from build123d import *

# Parameters (mm, degrees)
SK_TOP_PLATE_R         = 1.7
SK_TOP_PLATE_R_2       = 6
TOP_PLATE_DEPTH        = 10
SK_YAW_PILOT_RECESS_R  = 17.15
YAW_PILOT_RECESS_DEPTH = 2.2
SK_BACK_PLATE_W        = 132
SK_BACK_PLATE_H        = 100
SK_BACK_PLATE_R        = 2.25
SK_BACK_PLATE_R_2      = 13
BACK_PLATE_DEPTH       = 8
RIB_DEPTH              = 8


with BuildPart() as part:
    # SK_Top_Plate → Top_Plate (new body)
    with BuildSketch(Plane.XY.offset(72)):
        Polygon((-122, 45), (18, 45), (36, 27), (36, -27), (18, -45), (-122, -45), (-140, -27), (-140, 27), align=None)
        with Locations((23, 0)):
            Circle(SK_TOP_PLATE_R, mode=Mode.SUBTRACT)
        with Locations((11.5, -19.918584287)):
            Circle(SK_TOP_PLATE_R, mode=Mode.SUBTRACT)
        with Locations((-11.5, -19.918584287)):
            Circle(SK_TOP_PLATE_R, mode=Mode.SUBTRACT)
        with Locations((-23, 0)):
            Circle(SK_TOP_PLATE_R, mode=Mode.SUBTRACT)
        with Locations((-11.5, 19.918584287)):
            Circle(SK_TOP_PLATE_R, mode=Mode.SUBTRACT)
        with Locations((11.5, 19.918584287)):
            Circle(SK_TOP_PLATE_R, mode=Mode.SUBTRACT)
        Circle(SK_TOP_PLATE_R_2, mode=Mode.SUBTRACT)
    extrude(amount=TOP_PLATE_DEPTH)

    # SK_Yaw_Pilot_Recess → Yaw_Pilot_Recess (cut)
    with BuildSketch(Plane.XY.offset(82)):
        Circle(SK_YAW_PILOT_RECESS_R)
    extrude(amount=-YAW_PILOT_RECESS_DEPTH, mode=Mode.SUBTRACT)

    # SK_Back_Plate → Back_Plate (add)
    with BuildSketch(Plane(origin=(-140, 0, 0), x_dir=(0, 0, -1), z_dir=(1, 0, 0))):
        with Locations((-16, 0)):
            Rectangle(SK_BACK_PLATE_W, SK_BACK_PLATE_H)
        with Locations((39.726819898, -16.455387592)):
            Circle(SK_BACK_PLATE_R, mode=Mode.SUBTRACT)
        with Locations((16.455387592, -39.726819898)):
            Circle(SK_BACK_PLATE_R, mode=Mode.SUBTRACT)
        with Locations((-16.455387592, -39.726819898)):
            Circle(SK_BACK_PLATE_R, mode=Mode.SUBTRACT)
        with Locations((-39.726819898, -16.455387592)):
            Circle(SK_BACK_PLATE_R, mode=Mode.SUBTRACT)
        with Locations((-39.726819898, 16.455387592)):
            Circle(SK_BACK_PLATE_R, mode=Mode.SUBTRACT)
        with Locations((-16.455387592, 39.726819898)):
            Circle(SK_BACK_PLATE_R, mode=Mode.SUBTRACT)
        with Locations((16.455387592, 39.726819898)):
            Circle(SK_BACK_PLATE_R, mode=Mode.SUBTRACT)
        with Locations((39.726819898, 16.455387592)):
            Circle(SK_BACK_PLATE_R, mode=Mode.SUBTRACT)
        Circle(SK_BACK_PLATE_R_2, mode=Mode.SUBTRACT)
    extrude(amount=BACK_PLATE_DEPTH)

    # SK_Rib → Rib (add)
    with BuildSketch(Plane(origin=(0, -4, 0), x_dir=(1, 0, 0), z_dir=(0, 1, 0))):
        Polygon((-140, -52), (-30, -72), (-140, -72), align=None)
    extrude(amount=RIB_DEPTH)


solid = part.part
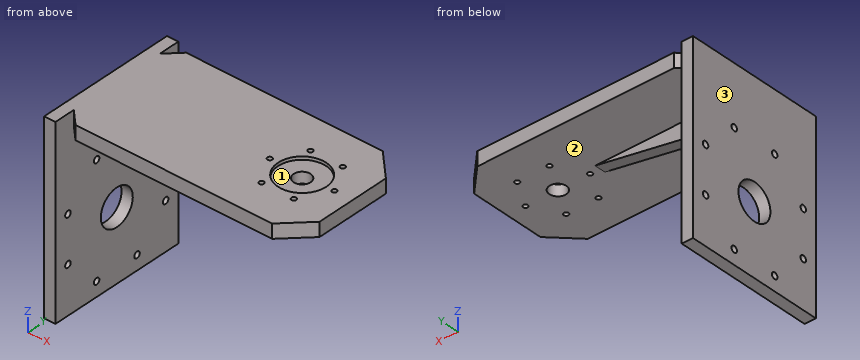
Work out the finished part from the listing and answer in its coordinate system (mm). Face numbers are marked on the shaded views. Give positions to 0.01 mm unless a question says otherwise; leave off trailing zeros. Loops run counter-clockwise (first coordinate to the right, second up) from the corner with the lowest first, then second, coordinate; pieces in that order, holes last. Notation, with made-up numbers: (17, 56) -> (25, 56) arc R19 cw to (25, 92) -> close; hole circle Ø7 at (-6, 33.25). An arc over 180 degrees is marked (long way). Use a Markdown table: item, result. Add a question column.
1. Flat-ended cylindrical pins translate along their axes: pin 1 Ø6 at (y, z) = (16.46, -39.73) entering from +X; pin 2 Ø6 at (x, y) = (-42.5, 1.5) entering from -Z; pin 3 Ø15.5 at (x, y) = (0, 0) entering from -Z. Find the tip coordinate at first contact, or state that the pin passes through.
2. Section C-C on z = 56 is taken. Determine the outline of the cut face in (x, y), and give its area (3 significant figures).
3. Section A-A on x = 0 is taken. Determine the outline of the cut face in (y, z), and give its area (3 significant figures).
4. Determine the mould class of the marked faces 1, 2 and 3 for opening direction X: released by +X, released by -X, zero draft, split by the parting line, or undercut.
5. Section B-B on z = 0 is taken. Determine the outline of the cut face in (x, y).
6. Find the intervals of material crossed by probe 1 along Y at (x, z) = (0, 78); probe 2 along X at (y, z) = (-15.5, -43); probe 3 along Z at (x, y) = (-41, 14), in increasing order.
7. Section D-D on x = -78 is taken. Determine the outline of the cut face in (y, z).
Results below:
| question | item | result |
|---|---|---|
| 1 | pin 1 | stops at x = -132 |
| 1 | pin 2 | stops at z = 69.18 |
| 1 | pin 3 | stops at z = 72 |
| 2 | outline | (-140, -50) -> (-132, -50) -> (-132, -4) -> (-118, -4) -> (-118, 4) -> (-132, 4) -> (-132, 50) -> (-140, 50) -> close |
| 2 | area | 912 mm^2 |
| 3 | outline | (-45, 72) -> (-6, 72) -> (-6, 79.8) -> (-17.15, 79.8) -> (-17.15, 82) -> (-45, 82) -> close; (6, 72) -> (45, 72) -> (45, 82) -> (17.15, 82) -> (17.15, 79.8) -> (6, 79.8) -> close |
| 3 | area | 731 mm^2 |
| 4 | face 1 | undercut |
| 4 | face 2 | zero draft |
| 4 | face 3 | released by -X |
| 5 | outline | (-140, -50) -> (-132, -50) -> (-132, -13) -> (-140, -13) -> close; (-140, 13) -> (-132, 13) -> (-132, 50) -> (-140, 50) -> close |
| 6 | probe 1 | y = -45 to -6, 6 to 45 |
| 6 | probe 2 | x = -140 to -132 |
| 6 | probe 3 | z = 72 to 82 |
| 7 | outline | (-45, 72) -> (-4, 72) -> (-4, 63.27) -> (4, 63.27) -> (4, 72) -> (45, 72) -> (45, 82) -> (-45, 82) -> close |
